```python
from build123d import *

# Parameters (mm, degrees)
F1_DEPTH = 5
F2_R     = 1.254284
F3_DEPTH = 25
F4_R     = 1.25
F5_DEPTH = 25


with BuildPart() as f1:
    # F0 (on Front) → F1 (new body)
    with BuildSketch(Plane.XZ):
        Polygon((-12.037362, -37.981261), (-12.037362, -32.436818), (12.962638, -32.436818), (12.962638, -37.981261), (17.962638, -37.981261), (21.440424, -15.064236), (21.440424, -10.040002), (12.962638, -10.040002), (12.962638, -5.040002), (-12.037362, -5.040002), (-12.037362, -10.040002), (-20.515148, -10.040002), (-20.515148, -15.064236), (-17.037362, -37.981261), align=None)
    extrude(amount=F1_DEPTH)

    # F2 (on face) → F3 (cut)
    with BuildSketch(Plane(origin=(12.962638, 0, 0), x_dir=(0, -1, 0), z_dir=(-1, 0, 0))):
        with Locations((2.5, -35.481261)):
            Circle(F2_R)
    extrude(amount=-F3_DEPTH, mode=Mode.SUBTRACT)

    # F4 (on face) → F5 (cut)
    with BuildSketch(Plane.YZ.offset(12.962638)):
        with Locations((-2.5, -7.540002)):
            Circle(F4_R)
    extrude(amount=-F5_DEPTH, mode=Mode.SUBTRACT)


solid = f1.part
```
Can you work these out from the model? Positions are in its coordinate system, mm. A direction names the side the tool comes from. Coordinates: 2 decimals unless noted, no trailing zeros. Write each loop counter-clockwise with the first axis right and the second up, starting at its lowest first coordinate (ties: lowest second). Pieces come first, ordered by that corner, then holes. Notation, with made-up numbers: M -30.5,76 L -9.5,76 A24 cw -9.5,104 Z; hole C -3,-11 d3. An arc over 180 degrees is marked long. Answer as CSV lines item,"result".
Item 1: We'd pull the mould along Y, two halves only. Please class faces 1 (the flat face through (0, 0, -21)), 2 (the cylindrical face through (0.638, -1.923, -8.649)), 3 (the flat face through (-12.037, -1, -7)), 4 (the flat face through (0, -5, -21)): +Y half, -Y half, draft (parallel to the pull), parting line (faces both ways), or undercut.
Geometry results:
face 1,"+Y half"
face 2,"undercut"
face 3,"draft"
face 4,"-Y half"
Item 2: Imagine slicing it at D-D on z = -9.5. List the corners of the cut face in (x, y) for me.
Geometry results:
outline,"M -12.04,-5 L 12.96,-5 L 12.96,0 L -12.04,0 Z"
Item 3: Please list where these lines run through material, in increasing order: line 1 along Z through (x, y) = (15.05, -2.5); line 2 along Z through (x, y) = (-1.75, -2.5); line 3 along X through (y, z) = (-4, -9.5).
Geometry results:
line 1,"z = -37.98 to -36.74, -34.23 to -10.04"
line 2,"z = -32.44 to -8.79, -6.29 to -5.04"
line 3,"x = -12.04 to 12.96"
Item 4: Imagine slicing it at C-C on y = -2.05. List the corners of the cut face in (x, z) for me.
Geometry results:
outline,"M -20.52,-15.06 L -17.04,-37.98 L -12.04,-37.98 L -12.04,-32.44 L 12.96,-32.44 L 12.96,-34.31 L 18.52,-34.31 L 21.44,-15.06 L 21.44,-10.04 L 12.96,-10.04 L 12.96,-8.71 L -12.04,-8.71 L -12.04,-10.04 L -20.52,-10.04 Z; M -12.04,-6.37 L 12.96,-6.37 L 12.96,-5.04 L -12.04,-5.04 Z; M 12.96,-37.98 L 17.96,-37.98 L 18.16,-36.65 L 12.96,-36.65 Z"
Item 5: I'm going to push flat-ended pins straight in: P1, Ø2.5, axis at x = -3.5, y = -3, coming from the -Z side; P2, Ø1.5, axis at y = -2.5, z = -35.48, coming from the +X side; P3, Ø2.5, axis at y = -3, z = -7, coming from the -X side. Where does each tip first touch, or does it pass through?
Geometry results:
P1,"stops at z = -32.44"
P2,"stops at x = -12.04"
P3,"stops at x = -12.04"
Item 6: On a 3-axis mill with a long thin cutter (end or side, diameter ignored), from which of +Z, -Z, +X, -X, +Y, -Y can I reach the whole of each face in a straight line? I mean faces 5 (the flat face through (-16, -2, -10.04)), 6 (the flat face through (12.963, -2, -34)), 7 (the flat face through (12.963, -1, -8)), 8 (the cylindrical face through (15.727, -2.337, -34.238)). Say none if no direction works.
Geometry results:
face 5,"+Z, -X, +Y, -Y"
face 6,"-Z, +Y, -Y"
face 7,"+Z, +X, +Y, -Y"
face 8,"+X"
Item 7: Imagine slicing it at A-A on y = -4.4. List the corners of the cut face in (x, z) for me.
Geometry results:
outline,"M -20.52,-15.06 L -17.04,-37.98 L -12.04,-37.98 L -12.04,-32.44 L 12.96,-32.44 L 12.96,-37.98 L 17.96,-37.98 L 21.44,-15.06 L 21.44,-10.04 L 12.96,-10.04 L 12.96,-5.04 L -12.04,-5.04 L -12.04,-10.04 L -20.52,-10.04 Z"
Item 8: Imagine slicing it at B-B on x = -5.5. List the corners of the cut face in (y, z) for me, plus the area to 3 significant figures.
Geometry results:
outline,"M -5,-32.44 L 0,-32.44 L 0,-5.04 L -5,-5.04 Z; hole C -2.5,-7.54 d2.5"
area,"132 mm2"
